Model file for the job. Use its own axes, mm. Face numbers are marked on the shaded views. A direction names the side the tool comes from. Give positions to 0.01 mm unless a question says otherwise; leave off trailing zeros. Write each loop counter-clockwise with the first axis right and the second up, starting at its lowest first coordinate (ties: lowest second). Pieces come first, ordered by that corner, then holes.
```python
from build123d import *

# Parameters (mm, degrees)
SKETCH_1_W           = 135
SKETCH_1_H           = 20
EXTRUDE_3_DEPTH      = 12
CUT_EXTRUDE_1_DEPTH  = 62.5
SKETCH_16_R          = 1.35
EXTRUDE_4_DEPTH      = 12
SKETCH_17_R          = 1.35
CUT_EXTRUDE_12_DEPTH = 81.779019553


with BuildPart() as part:
    # 草图1 → 凸台-拉伸3 (new body)
    with BuildSketch(Plane(origin=(0, 0, 0), x_dir=(1, 0, 0), z_dir=(0, 1, 0))):
        Rectangle(SKETCH_1_W, SKETCH_1_H)
    extrude(amount=EXTRUDE_3_DEPTH)

    # 草图2 → 切除-拉伸1 (cut, symmetric)
    with BuildSketch(Plane(origin=(0, 0, 0), x_dir=(0, 0, -1), z_dir=(1, 0, 0))):
        Polygon((-7.5, 12), (-2.5, 3), (-2.5, 0), (2.5, 0), (2.5, 3), (7.5, 12), align=None)
    extrude(amount=CUT_EXTRUDE_1_DEPTH, both=True, mode=Mode.SUBTRACT)

    # 草图16 → 凸台-拉伸4 (add)
    with BuildSketch(Plane(origin=(0, 12, 0), x_dir=(1, 0, 0), z_dir=(0, 1, 0))):
        Polygon((60.5, 10), (67.5, 10), (67.5, -10), (68.5, -10), (68.5, 0), (76.5, 0), (76.5, 13), (60.5, 13), align=None)
        with Locations(Location((69.5, 9, 0), (0, 0, 270))):
            Circle(SKETCH_16_R, mode=Mode.SUBTRACT)
    extrude(amount=-EXTRUDE_4_DEPTH)

    # 草图17 → 切除-拉伸12 (cut, through all)
    with BuildSketch(Plane(origin=(0, 0, -13), x_dir=(-1, 0, 0), z_dir=(0, 0, -1))):
        with Locations((-65.5, 6)):
            Circle(SKETCH_17_R)
        with Locations((-73.5, 6)):
            Circle(SKETCH_17_R)
    extrude(amount=-CUT_EXTRUDE_12_DEPTH, mode=Mode.SUBTRACT)


solid = part.part
```
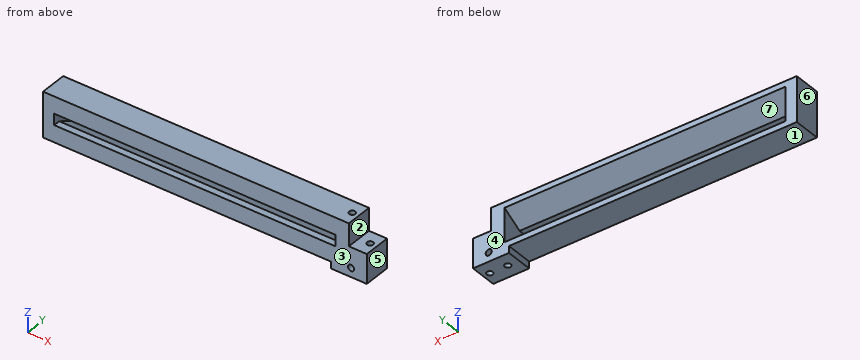
1. Pull direction X, two halves, no side cores. Call the marked faces 4, 5, 6 and 7: +X half, -X half, draft (parallel to the pull), parting line (faces both ways), or undercut.
Calculated:
face 4: draft
face 5: +X half
face 6: -X half
face 7: undercut
2. Slice it at A-A, the plane x = 52. Write the cut outline in (y, z), and give its area (3 significant figures).
Calculated:
outline: (0, -10) - (12, -10) - (12, -7.5) - (3, -2.5) - (0, -2.5) - close; (0, 2.5) - (3, 2.5) - (12, 7.5) - (12, 10) - (0, 10) - close
area: 135 mm2
3. Probe probe 1 along Y at (x, z) = (65.5, -0.25); probe 2 along X at (y, z) = (5, -9); probe 3 along Z at (x, y) = (-27, 1.75). List the from-to ranges inside material, lowest first.
Calculated:
probe 1: y = 0 to 4.65, 7.35 to 12
probe 2: x = -67.5 to 64.59, 66.41 to 68.15, 70.85 to 72.59, 74.41 to 76.5
probe 3: z = -10 to -2.5, 2.5 to 10
4. Pin check, flat tips, straight feed: P1, Ø2, axis at x = 73.5, y = 6, coming from the +Z side; P2, Ø3.5, axis at x = -9, y = 1, coming from the -Z side; P3, Ø0.9, axis at y = 6.5, z = -11, coming from the -X side; P4, Ø2, axis at y = 4.5, z = 3, coming from the +X side. Stop position of each tip, or through.
Calculated:
P1: passes through
P2: stops at z = -10
P3: stops at x = 60.5
P4: stops at x = 68.5
5. Which spindle directions (+Z, -Z, +X, -X, +Y, -Y) get a long thin tool onto all of the face, cutting with end or side? Do the marked faces 1, 2 and 3. Say none if no direction does.
Calculated:
face 1: -Z, -X, +Y, -Y
face 2: +Z, +X, +Y, -Y
face 3: +Z, -Z, +X, -X, -Y
6. Slice it at C-C, the plane y = 6. Write the cut outline in (x, z), and give its area (3 significant figures).
Calculated:
outline: (-67.5, -10) - (60.5, -10) - (60.5, -13) - (64.15, -13) - (64.15, 10) - (-67.5, 10) - close; (66.85, -13) - (72.15, -13) - (72.15, 0) - (68.5, 0) - (68.5, 10) - (66.85, 10) - close; (74.85, -13) - (76.5, -13) - (76.5, 0) - (74.85, 0) - close; hole (-62.5, -4.17) - (62.5, -4.17) - (62.5, 4.17) - (-62.5, 4.17) - close; hole circle Ø2.7 at (69.5, -9)
area: 1,700 mm2
7. Slice it at B-B, the plane z = -4.5. Write the cut outline in (x, y), and give its area (3 significant figures).
Calculated:
outline: (-67.5, 0) - (76.5, 0) - (76.5, 12) - (62.5, 12) - (62.5, 6.6) - (-62.5, 6.6) - (-62.5, 12) - (-67.5, 12) - close; hole circle Ø2.7 at (65.5, 6); hole circle Ø2.7 at (73.5, 6)
area: 1,040 mm2
